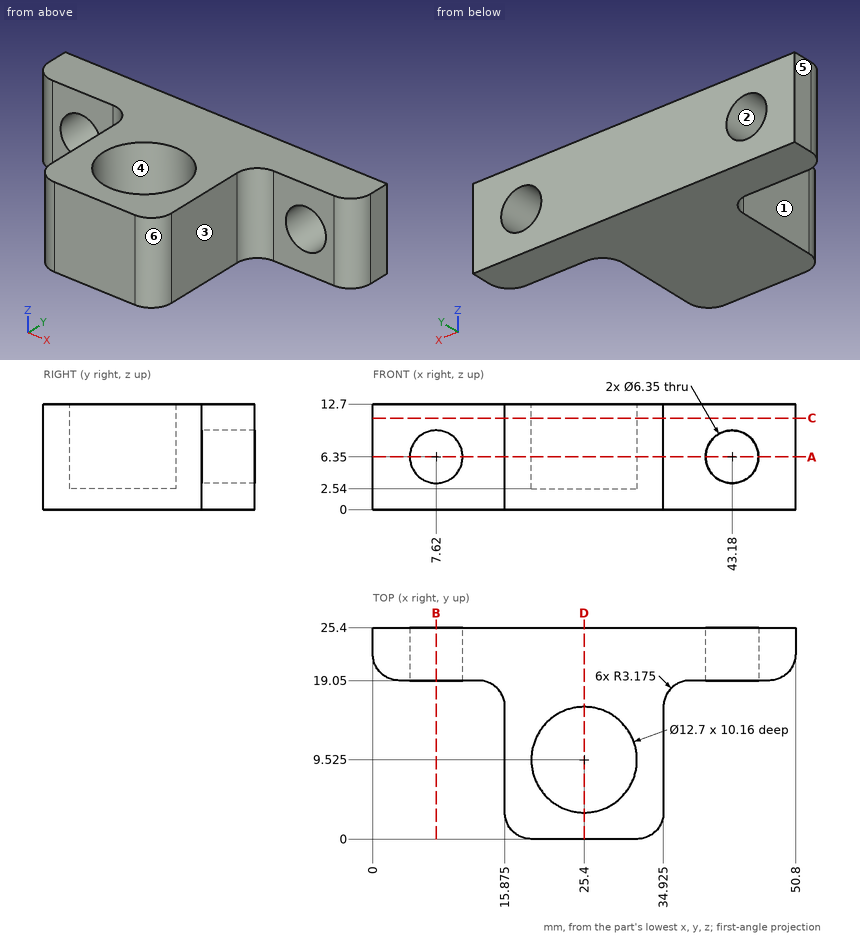
Check sheet for the drawn part. Datum: minimum x, y, z corner. Units: mm. A direction names the side the tool comes from. Round coordinates to 2 decimals unless told otherwise and drop trailing zeros. Loops run counter-clockwise (first coordinate to the right, second up) from the corner with the lowest first, then second, coordinate; pieces in that order, holes last. Notation, with made-up numbers: (-4.75, 71.5) - (48.25, 71.5) arc R26 cw to (48.25, 105.5) - close; hole circle Ø11 at (7.25, 57.5). An arc over 180 degrees is marked (long way). Answer as a JSON object with one key per item and string values. Group by question number.
Q1. Sectioned sample at C-C, the plane z = 11. Enter the section's corners in (x, y) (3 decimals).
Q2. Gauge pin test, flat ends, axial feed: P1, Ø3, axis at y = 3.5, z = 5, coming from the +X side (3 decimals); P2, Ø7.5, axis at x = 7.62, z = 6.35, coming from the -Y side; P3, Ø3, axis at y = 19, z = 9, coming from the -X side; P4, Ø5.5, axis at x = 43.18, z = 6.35, coming from the +Y side. Record the tip position at first contact, or that the pin passes through.
Q3. Mould release check, pull along Y, two halves, no side actions. Record for the marked faces 4, 5 and 6: released by +Y, released by -Y, zero draft, split by the parting line, or undercut.
Q4. Scan lines: line 1 along Z through (x, y) = (20, 6.5); line 2 along Y through (x, z) = (22.5, 11); line 3 along Z through (x, y) = (7.62, 21) (3 decimals). Record each from-to range of solid material in increasing order. Write a range as [from, to].
Q5. Set-up check for the marked faces 1, 2 and 3: record each of +Z, -Z, +X, -X, +Y, -Y from which the full face is reachable in a straight line by a thin tool's end or side.
Q6. Sectioned sample at A-A, the plane z = 6.35. Enter the section's corners in (x, y) (3 decimals), plus the area to 3 significant figures.
Q7. Sectioned sample at D-D, the plane x = 25.4. Enter the section's corners in (y, z) (3 decimals), plus the area to 3 significant figures.
Q8. Sectioned sample at B-B, the plane x = 7.62. Enter the section's corners in (y, z) (3 decimals).
Solution:
{
 "1": {"outline": "(0, 22.225) arc R3.175 ccw to (3.175, 19.05) - (12.7, 19.05) arc R3.175 cw to (15.875, 15.875) - (15.875, 3.175) arc R3.175 ccw to (19.05, 0) - (31.75, 0) arc R3.175 ccw to (34.925, 3.175) - (34.925, 15.875) arc R3.175 cw to (38.1, 19.05) - (47.625, 19.05) arc R3.175 ccw to (50.8, 22.225) - (50.8, 25.4) - (0, 25.4) - close; hole circle Ø12.7 at (25.4, 9.525)"},
 "2": {"P1": "stops at x = 34.925", "P2": "stops at y = 19.05", "P3": "stops at x = 0.51", "P4": "passes through"},
 "3": {"face 4": "undercut", "face 5": "zero draft", "face 6": "released by -Y"},
 "4": {"line 1": "z = [0, 2.54]", "line 2": "y = [0, 3.88], [15.17, 25.4]", "line 3": "z = [0, 3.175], [9.525, 12.7]"},
 "5": {"face 1": "+Z, -Z, -X, -Y", "face 2": "+Y, -Y", "face 3": "+Z, -Z, +X, -Y"},
 "6": {"outline": "(0, 22.225) arc R3.175 ccw to (3.175, 19.05) - (4.445, 19.05) - (4.445, 25.4) - (0, 25.4) - close; (10.795, 19.05) - (12.7, 19.05) arc R3.175 cw to (15.875, 15.875) - (15.875, 3.175) arc R3.175 ccw to (19.05, 0) - (31.75, 0) arc R3.175 ccw to (34.925, 3.175) - (34.925, 15.875) arc R3.175 cw to (38.1, 19.05) - (40.005, 19.05) - (40.005, 25.4) - (10.795, 25.4) - close; (46.355, 19.05) - (47.625, 19.05) arc R3.175 ccw to (50.8, 22.225) - (50.8, 25.4) - (46.355, 25.4) - close; hole circle Ø12.7 at (25.4, 9.525)", "area": "474 mm²"},
 "7": {"outline": "(0, 0) - (25.4, 0) - (25.4, 12.7) - (15.875, 12.7) - (15.875, 2.54) - (3.175, 2.54) - (3.175, 12.7) - (0, 12.7) - close", "area": "194 mm²"},
 "8": {"outline": "(19.05, 0) - (25.4, 0) - (25.4, 3.175) - (19.05, 3.175) - close; (19.05, 9.525) - (25.4, 9.525) - (25.4, 12.7) - (19.05, 12.7) - close"}
}
